from build123d import *

# Parameters (mm, degrees)
SKETCH_1_W          = 40
SKETCH_1_H          = 80
EXTRUDE_1_DEPTH     = 15
SKETCH_2_R          = 8.05
CUT_EXTRUDE_1_DEPTH = 60
SKETCH_3_W          = 25
SKETCH_3_H          = 16.969379431
CUT_EXTRUDE_2_DEPTH = 60
SKETCH_4_R          = 1.45
CUT_EXTRUDE_3_DEPTH = 35
CUT_EXTRUDE_4_DEPTH = 35
FILLET_1_R          = 2


with BuildPart() as part:
    # 草图1 → 凸台-拉伸1 (new body)
    with BuildSketch(Plane.XY):
        Rectangle(SKETCH_1_W, SKETCH_1_H)
    extrude(amount=EXTRUDE_1_DEPTH)

    # 草图2 → 切除-拉伸1 (cut)
    with BuildSketch(Plane.XY.offset(15)):
        with Locations((0, 20)):
            Circle(SKETCH_2_R)
    extrude(amount=-CUT_EXTRUDE_1_DEPTH, mode=Mode.SUBTRACT)

    # 草图3 → 切除-拉伸2 (cut)
    with BuildSketch(Plane.XY.offset(15)):
        with Locations((0, -36.484689715)):
            Rectangle(SKETCH_3_W, SKETCH_3_H)
    extrude(amount=-CUT_EXTRUDE_2_DEPTH, mode=Mode.SUBTRACT)

    # 草图4 → 切除-拉伸3 (cut)
    with BuildSketch(Plane.XZ.offset(28)):
        with Locations(Location((0, 7.5, 0), (0, 0, 270))):
            Circle(SKETCH_4_R)
    extrude(amount=-CUT_EXTRUDE_3_DEPTH, mode=Mode.SUBTRACT)

    # 草图5 → 切除-拉伸4 (cut)
    with BuildSketch(Plane.XY.offset(15)):
        with BuildLine():
            Line((-7.5, 5), (-7.5, -17))
            ThreePointArc((-7.5, -17), (-11, -20.5), (-14.5, -17))
            Line((-14.5, -17), (-14.5, 5))
            ThreePointArc((-14.5, 5), (-11, 8.5), (-7.5, 5))
        make_face()
        with BuildLine():
            Line((14.5, 5), (14.5, -17))
            ThreePointArc((14.5, -17), (11, -20.5), (7.5, -17))
            Line((7.5, -17), (7.5, 5))
            ThreePointArc((7.5, 5), (11, 8.5), (14.5, 5))
        make_face()
    extrude(amount=-CUT_EXTRUDE_4_DEPTH, mode=Mode.SUBTRACT)

    # 圆角1
    fillet_1_edges = [part.edges().sort_by_distance(p)[0] for p in [
        (12.5, -28, 7.5),
        (-12.5, -28, 7.5),
        (-20, 40, 7.5),
        (20, 40, 7.5),
    ]]
    fillet(fillet_1_edges, radius=FILLET_1_R)


solid = part.part
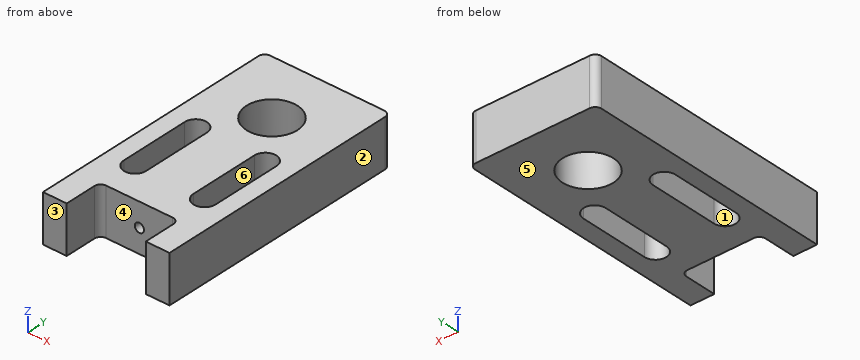
Input: part model. Units: mm. Frame: model coordinates. Face numbers are marked on the shaded views. A direction names the side the tool comes from. Give positions to 0.01 mm unless a question says otherwise; leave off trailing zeros. Order: outer loops, then holes, each group sorted by start corner. A loop starts at its lowest first (then second) coordinate and runs counter-clockwise, first axis right, second up.
Q1. Section A-A on x = 0. Output: boundary loops of the cut face in (y, z), and give its area (3 significant figures).
Checked values:
outline: (-28, 0) - (11.95, 0) - (11.95, 15) - (-28, 15) - (-28, 8.95) - (7, 8.95) - (7, 6.05) - (-28, 6.05) - close; (28.05, 0) - (40, 0) - (40, 15) - (28.05, 15) - close
area: 677 mm2
Q2. Section B-B on y = 20. Output: boundary loops of the cut face in (x, z), and give its area (4 significant figures).
Checked values:
outline: (-20, 0) - (-8.05, 0) - (-8.05, 15) - (-20, 15) - close; (8.05, 0) - (20, 0) - (20, 15) - (8.05, 15) - close
area: 358.5 mm2
Q3. Section C-C on z = 12.5. Output: boundary loops of the cut face in (x, y).
Checked values:
outline: (-20, -40) - (-12.5, -40) - (-12.5, -30) arc R2 cw to (-10.5, -28) - (10.5, -28) arc R2 cw to (12.5, -30) - (12.5, -40) - (20, -40) - (20, 38) arc R2 ccw to (18, 40) - (-18, 40) arc R2 ccw to (-20, 38) - close; hole (-14.5, -17) arc R3.5 ccw to (-7.5, -17) - (-7.5, 5) arc R3.5 ccw to (-14.5, 5) - close; hole circle Ø16.1 at (0, 20); hole (7.5, -17) arc R3.5 ccw to (14.5, -17) - (14.5, 5) arc R3.5 ccw to (7.5, 5) - close
Q4. Section D-D on y = -3. Output: boundary loops of the cut face in (x, z), and give its area (3 significant figures).
Checked values:
outline: (-20, 0) - (-14.5, 0) - (-14.5, 15) - (-20, 15) - close; (-7.5, 0) - (7.5, 0) - (7.5, 15) - (-7.5, 15) - close; (14.5, 0) - (20, 0) - (20, 15) - (14.5, 15) - close; hole circle Ø2.9 at (0, 7.5)
area: 383 mm2
Q5. Set-up query: the marked faces 4, 5 and 6. Return all of +Z, -Z, +X, -X, +Y, -Y with unobstructed straight access to the full face (end or side cutting, diameter ignored); none if empty.
Checked values:
face 4: +Z, -Z, -Y
face 5: -Z, +X, -X, +Y, -Y
face 6: +Z, -Z
Q6. Ray query, probe 1 along X at (y, z) = (-5.5, 7.5); probe 2 along Y at (x, z) = (0, 10.5); probe 3 along X at (y, z) = (-19, 7.5). Return the intervals inside material, ascending.
Checked values:
probe 1: x = -20 to -14.5, -7.5 to -1.45, 1.45 to 7.5, 14.5 to 20
probe 2: y = -28 to 11.95, 28.05 to 40
probe 3: x = -20 to -13.87, -8.13 to -1.45, 1.45 to 8.13, 13.87 to 20
Q7. Contact query for flat-ended pins moving along their axis: pin 1 Ø0.9 at (x, z) = (-0.5, 7.5) entering from -Y; pin 2 Ø1 at (x, y) = (-9, -14) entering from -Z. Output: stop coordinate, or through.
Checked values:
pin 1: stops at y = 7
pin 2: passes through
Q8. Draft query along X for the marked faces 1, 2 and 3. Return one class per face: +X half, -X half, draft (parallel to the pull), parting line (faces both ways), or undercut.
Checked values:
face 1: undercut
face 2: +X half
face 3: draft
